Autodesk Inventor part; units mm, degrees
ref_plane "YZ Plane" through (0, 0, 0) normal (1, 0, 0) x (0, 1, 0)
ref_plane "XZ Plane" through (0, 0, 0) normal (0, 1, 0) x (-1, 0, 0)
ref_plane "XY Plane" through (0, 0, 0) normal (0, 0, 1) x (1, 0, 0)
sketch "Sketch1" plane through (0, 0, 0) normal (0, 1, 0) x (-1, 0, 0)
  line L0 (-74.75, 42.075) -> (74.75, 42.075)
  line L1 (74.75, 42.075) -> (74.75, -42.075)
  line L2 (74.75, -42.075) -> (-74.75, -42.075)
  line L3 (-74.75, -42.075) -> (-74.75, 42.075)
  line L4 (-74.75, 42.075) -> (74.75, -42.075) construction
  line L5 (74.75, 42.075) -> (-74.75, -42.075) construction
  point P0 (0, 0)
  dimension "d0" = 149.5
  dimension "d1" = 84.15
extrude "Extrusion1" add sketch "Sketch1" along normal blind 4.064
sketch "Sketch2" plane through (0, 4.064, 0) normal (0, 1, 0) x (1, 0, 0)
  point P0 (0, 0)
  point P1 (-60, 30)
  point P2 (60, 30)
  point P3 (-60, -30)
  point P4 (60, -30)
  dimension "d4" = 60
  dimension "d5" = 30
  dimension "d6" = 60
  dimension "d7" = 30
  dimension "d8" = 30
  dimension "d9" = 60
  dimension "d10" = 30
  dimension "d11" = 60
hole "Hole1" at (-60, 4.064, -30) at (60, 4.064, -30) at (-60, 4.064, 30) at (60, 4.064, 30) direction (0, -1, 0) diameter 4.5 end through all countersink diameter 9.4 countersink angle 90
properties part number "Piston Feed Surface" material "Aluminum 6061"
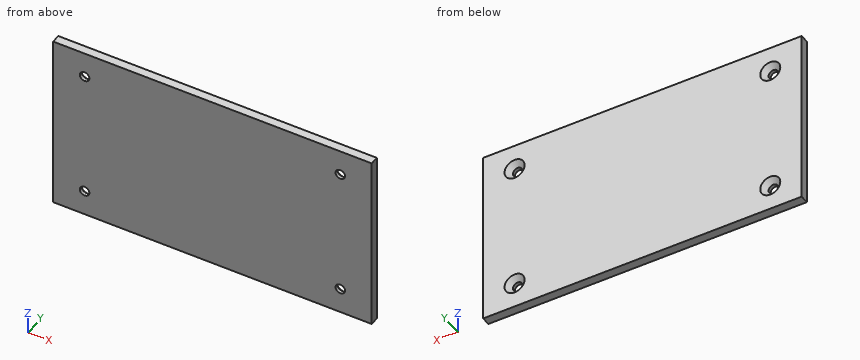
The listing builds one solid part. Answer for the finished solid, in the listing's coordinates (mm). Coordinates: 2 decimals unless noted, no trailing zeros. Loops run counter-clockwise (first coordinate to the right, second up) from the corner with the lowest first, then second, coordinate; pieces in that order, holes last. Notation, with made-up numbers: M 48,78.5 L 99,78.5 A18 ccw 99,103.5 Z; hole C -33.5,-2.75 d5. An arc over 180 degrees is marked long. Answer as a JSON object with one key per item and string values. Group by question number.
Item 1: Section A-A (z = -30) is taken. Write down the section's boundary in (x, y), and give its area (3 significant figures).
Item 2: Consider L1, parallel to Z at x = -60, y = 0.8 (3 decimals); L2, parallel to X at y = 0.35, z = -30; L3, parallel to X at y = 3.05, z = 28. Determine where each line is inside the solid, lowest interval first.
Item 3: Each of these flat-tipped pins is pushed along its axis until it touches: P1, Ø4, axis at x = -60, z = -30, coming from the +Y side; P2, Ø5, axis at x = 60, z = -30, coming from the +Y side; P3, Ø7, axis at x = 60, z = 30, coming from the +Y side. Where does it stop, or does it pass through?
Item 4: Section B-B (x = -60) is taken. Write down the section's boundary in (y, z) (3 decimals), and give its area (3 significant figures).
Solved:
{
 "1": {"outline": "M -74.75,0 L -62.25,0 L -62.25,1.61 L -64.7,4.06 L -74.75,4.06 Z; M -57.75,0 L 57.75,0 L 57.75,1.61 L 55.3,4.06 L -55.3,4.06 L -57.75,1.61 Z; M 62.25,0 L 74.75,0 L 74.75,4.06 L 64.7,4.06 L 62.25,1.61 Z", "area": "559 mm2"},
 "2": {"L1": "z = -42.075 to -32.25, -27.75 to 27.75, 32.25 to 42.075", "L2": "x = -74.75 to -62.25, -57.75 to 57.75, 62.25 to 74.75", "L3": "x = -74.75 to -63.1, -56.9 to 56.9, 63.1 to 74.75"},
 "3": {"P1": "passes through", "P2": "stops at y = 1.86", "P3": "stops at y = 2.86"},
 "4": {"outline": "M 0,-42.075 L 4.064,-42.075 L 4.064,-34.7 L 1.614,-32.25 L 0,-32.25 Z; M 0,-27.75 L 1.614,-27.75 L 4.064,-25.3 L 4.064,25.3 L 1.614,27.75 L 0,27.75 Z; M 0,32.25 L 1.614,32.25 L 4.064,34.7 L 4.064,42.075 L 0,42.075 Z", "area": "293 mm2"}
}
